The listing builds one solid part. Answer for the finished solid, in the listing's coordinates (mm). A direction names the side the tool comes from. Coordinates: 2 decimals unless noted, no trailing zeros. Order: outer loops, then holes, each group sorted by start corner. A loop starts at its lowest first (then second) coordinate and runs counter-clockwise, first axis right, second up. Notation, with made-up numbers: M 72,-29 L 116,-29 A21 cw 116,-3 Z; hole C -28,67 d10. An arc over 180 degrees is marked long. One line per item, written item: value. Start each with the question number.
Q1. Each of these flat-tipped pins is pushed along its axis until it touches: pin 1 Ø4 at (x, y) = (-34.5, -6) entering from +Z; pin 2 Ø2 at (x, y) = (-45.5, -13) entering from +Z; pin 3 Ø8 at (x, y) = (-27, -14.5) entering from -Z. Where does it stop, or does it pass through?
Q2. For faces 4 (the flat face through (-28, 0, 9)), 5 (the flat face through (-28, -2.54, 10)), determine the directions among +Z, -Z, +X, -X, +Y, -Y from which every point of the face is accessible in a straight line to the end or side of a thin tool.
Q3. The part is cut by section C-C on x = -37.5. Give the vertices of the cut face in (y, z), then the cut area to 3 significant figures.
Q4. The part is cut by section D-D on y = -1.75. Give the vertices of the cut face in (x, z), then the cut area to 3 significant figures.
Q5. The part is cut by section A-A on y = -23.25. Give the vertices of the cut face in (x, z), then the cut area to 3 significant figures.
Q6. The part is cut by section B-B on z = 3. Give the vertices of the cut face in (x, y), then the cut area to 3 significant figures.
Q7. Straight lines are drawn through the part: line 1 along Y through (x, z) = (-16.5, 13); line 2 along Z through (x, y) = (-44, -24); line 3 along Z through (x, y) = (-33, -12.75). For each, find the intervals that lie inside material, in ascending order. Write a range as [from, to].
Q8. Determine the mould class of faces 1 (the cylindrical face through (-6.88, -12.52, 2.8)), 2 (the flat face through (-27.98, -13.81, 0.308)), 3 (the flat face through (-40.2, -12.5, 17)) for opening direction Z: pulls with the +Z half, pulls with the -Z half, needs draft (parallel to the pull), parting line crosses it, or undercut.
```python
from build123d import *

# Parameters (mm, degrees)
F1_DEPTH = 25.4
F2_T     = -2.54
F3_R     = 3.81
F4_DEPTH = 19.05


# Not quite as in the source:
# - the program builds the solid bodies; features that only make, move or delete a surface that nothing else refers to are left out


with BuildPart() as f1:
    # F0 (on Front) → F1 (new body)
    with BuildSketch(Plane.XZ):
        with BuildLine():
            ThreePointArc((-12.1858643886, -0.9756983319), (-6.8419002324, 2.8860613911), (-7.8055765775, 9.4085202038))
            Line((-7.8055765775, 9.4085202038), (-22.3667159803, 26.9599173237))
            ThreePointArc((-22.3667159803, 26.9599173237), (-27.2929398052, 29.2553210157), (-32.1905035986, 26.8993863451))
            Line((-32.1905035986, 26.8993863451), (-48.3822646253, 6.8856646257))
            ThreePointArc((-48.3822646253, 6.8856646257), (-49.0625660789, -0.0700213051), (-42.9387648181, -3.4380229313))
            Line((-42.9387648181, -3.4380229313), (-12.1858643886, -0.9756983319))
        make_face()
    extrude(amount=F1_DEPTH)

    # F2
    f2_openings = [f1.faces().sort_by_distance(p)[0] for p in [
        (-28.02144, -25.4, 9.948419),
    ]]
    offset(amount=F2_T, openings=f2_openings)

    # F3 (on face) → F4 (join)
    with BuildSketch(Plane.XZ.offset(2.54)):
        with Locations((-43.4455749435, 2.8917198357)):
            Circle(F3_R)
    extrude(amount=F4_DEPTH)


solid = f1.part
```
Output:
1. pin 1: stops at z = 26.52
1. pin 2: stops at z = 11.68
1. pin 3: stops at z = -2.48
2. face 4: +Z, -Z, +X, -X, +Y
2. face 5: -Y
3. outline: M -25.4,-3 L 0,-3 L 0,20.34 L -25.4,20.34 L -25.4,16.3 L -2.54,16.3 L -2.54,-0.45 L -25.4,-0.45 Z
3. area: 210 mm^2
4. outline: M -48.38,6.89 A6.35 ccw -42.94,-3.44 L -12.19,-0.98 A6.35 ccw -7.81,9.41 L -22.37,26.96 A6.35 ccw -32.19,26.9 Z
4. area: 919 mm^2
5. outline: M -48.38,6.89 A6.35 ccw -42.94,-3.44 L -12.19,-0.98 A6.35 ccw -7.81,9.41 L -22.37,26.96 A6.35 ccw -32.19,26.9 Z; hole M -46.41,5.29 A3.81 ccw -43.14,-0.91 L -12.39,1.56 A3.81 ccw -9.76,7.79 L -24.32,25.34 A3.81 ccw -30.22,25.3 Z
5. area: 283 mm^2
6. outline: M -49.79,-25.4 L -47.25,-25.4 L -47.25,-21.59 L -39.64,-21.59 L -39.64,-2.54 L -9.7,-2.54 L -9.7,-25.4 L -6.8,-25.4 L -6.8,0 L -49.79,0 Z
6. area: 379 mm^2
7. line 1: y = [-2.54, 0]
7. line 2: z = [-3.43, -0.88], [8.26, 12.3]
7. line 3: z = [-2.64, -0.09], [21.86, 25.9]
8. face 1: parting line crosses it
8. face 2: undercut
8. face 3: pulls with the +Z half
